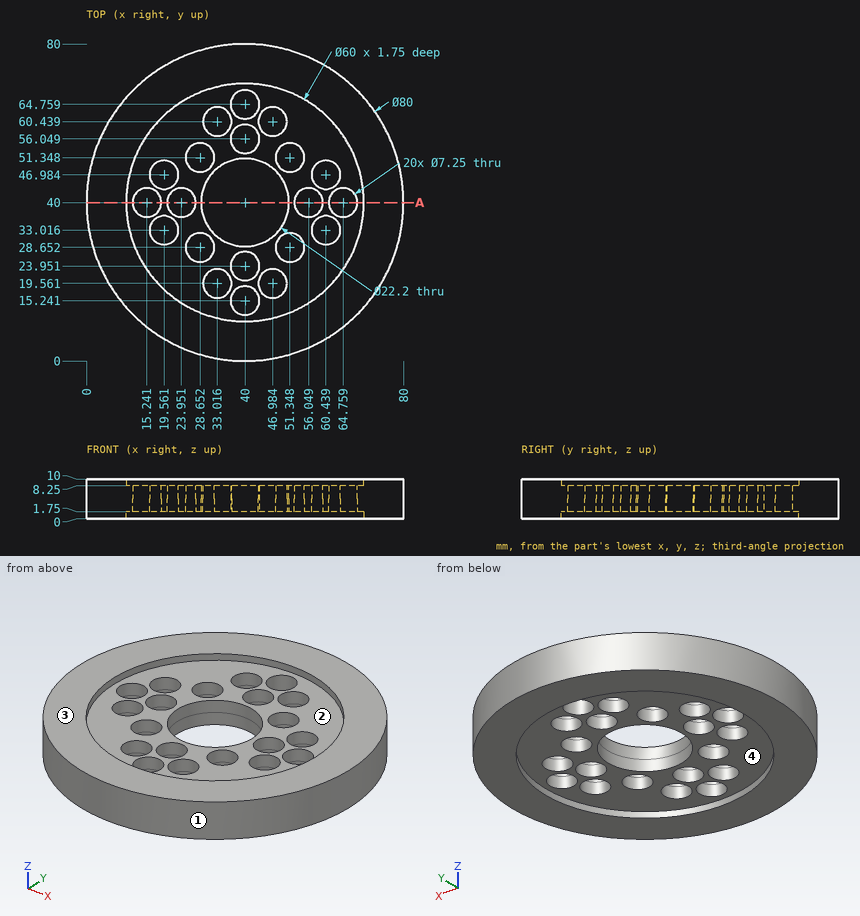
Part print with two shaded views. Sizes in mm from the minimum x, y, z corner. Round coordinates to 2 decimals unless told otherwise and drop trailing zeros. Use one line per item in the form item = value.
Item 1: Drill centre lines: line 1 (Y direction, x = 40, z = 2.5); line 2 (Y direction, x = 25.5, z = 3) (1 decimal); line 3 (X direction, y = 20, z = 7) (1 decimal). Where is each one in solid material? Low to high.
Returned:
line_1 = 0 to 11.62, 18.87 to 20.33, 27.58 to 28.9, 51.1 to 52.42, 59.67 to 61.13, 68.38 to 80
line_2 = 2.7 to 26.9, 30.4 to 36.7, 43.3 to 49.6, 53.1 to 77.3
line_3 = 5.4 to 29.4, 36.6 to 43.4, 50.6 to 74.6
Item 2: Pull direction X, two halves, no side cores. Call the marked faces 1, 2, 3 and 4: released by +X, released by -X, zero draft, split by the parting line, or undercut.
Returned:
face_1 = split by the parting line
face_2 = undercut
face_3 = zero draft
face_4 = undercut
Item 3: Flat gauge pins, fed straight in: pin 1 Ø4.5 at (x, y) = (15.24, 40) entering from -Z; pin 2 Ø8.5 at (x, y) = (60.44, 46.98) entering from +Z; pin 3 Ø2 at (x, z) = (38, 4.5) entering from -Y; pin 4 Ø3 at (y, z) = (25, 3) entering from +X. Where does each tip first touch, or does it go through?
Returned:
pin_1 = through
pin_2 = 8.25
pin_3 = 0.01
pin_4 = 77.65
Item 4: Cut at A-A, the plane y = 40. Give the number of separate pieces and of enclosed holes in the cut face, and give its area (3 significant figures).
Returned:
separate_pieces = 6
enclosed_holes = 0
area = 257 mm^2
